Geometry: final body of the model. Coordinates: model frame, mm. Give positions to 0.01 mm unless a question says otherwise; leave off trailing zeros. Order: outer loops, then holes, each group sorted by start corner. A loop starts at its lowest first (then second) coordinate and runs counter-clockwise, first axis right, second up. Notation, with made-up numbers: (70.5, 8) - (114.5, 8) arc R7 cw to (114.5, 14) - close; hole circle Ø9 at (38, 6.25). An arc over 180 degrees is marked (long way). Write item = value, one per line. Start each with the question number.
from build123d import *

# Parameters (mm, degrees)
F1_DEPTH = 50.8
F3_R     = 4.7625
F4_DEPTH = 12.7
F5_R     = 4.7625
F6_DEPTH = 9.525


with BuildPart() as f1:
    # F0 (on Front) → F1 (new body)
    with BuildSketch(Plane.XZ):
        Polygon((831.85, 9.525), (831.85, 19.05), (0, 19.05), (0, 0), (781.05, 0), (781.05, 9.525), align=None)
    extrude(amount=F1_DEPTH)

    # F3 (on offset) → F4 (cut, symmetric)
    with BuildSketch(Plane.XY.offset(9.525)):
        with Locations((806.45, -25.4)):
            Circle(F3_R)
        with Locations((581.025, -25.4)):
            Circle(F3_R)
    extrude(amount=F4_DEPTH, both=True, mode=Mode.SUBTRACT)

    # F5 (on Right) → F6 (join)
    with BuildSketch(Plane.YZ):
        with Locations((-25.4, 9.525)):
            Circle(F5_R)
    extrude(amount=-F6_DEPTH)


solid = f1.part
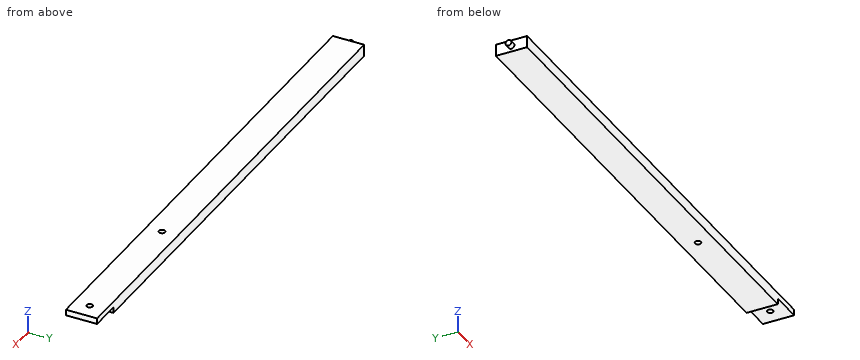
Q1. Contact query for flat-ended pins moving along their axis: pin 1 (7.5 mm diameter, centred on x = 806.45, y = -25.4, fed in from +Z); pin 2 (3 mm diameter, centred on y = -42.5, z = 10, fed in from -X). Output: stop coordinate, or through.
Q2. Section A-A, the plane y = -37. Return the cut outline in (x, z) (3 decimals).
Q3. Material intervals for line 1 along X through (y, z) = (-29, 10.5) (3 decimals); line 2 along X through (y, z) = (-27, 13.25) (3 decimals); line 3 along X through (y, z) = (-2.5, 16.5), sorted ascending. Write a range as from..to.
The answers:
q1.pin_1 = through
q1.pin_2 = 0
q2.outline = (0, 0) - (781.05, 0) - (781.05, 9.525) - (831.85, 9.525) - (831.85, 19.05) - (0, 19.05) - close
q3.line_1 = -9.525..577.907, 584.143..803.332, 809.568..831.85
q3.line_2 = -9.525..576.539, 585.511..801.964, 810.936..831.85
q3.line_3 = 0..831.85
